Input: part model. Units: mm. Frame: model coordinates. Face numbers are marked on the shaded views. A direction names the side the tool comes from. Coordinates: 2 decimals unless noted, no trailing zeros. Write each loop counter-clockwise with the first axis right and the second up, starting at its lowest first coordinate (ties: lowest second). Pieces come first, ordered by that corner, then holes. Notation, with made-up numbers: M 17.25,80.25 L 54.25,80.25 A18 cw 54.25,97.25 Z; hole C 36,63.25 d2. An arc over 180 degrees is marked long. Use one line per item in the form item = value.
from build123d import *

# Parameters (mm, degrees)
SKETCH5_R                = 20
BOSS_EXTRUDE2_DEPTH      = 15
SKETCH6_W                = 30
SKETCH6_H                = 90
BOSS_EXTRUDE3_DEPTH      = 15
CIRPATTERN1_COUNT        = 3
BOSS_EXTRUDE4_DEPTH      = 5
FILLET1_R                = 3
SKETCH8_R                = 1
CUT_EXTRUDE1_DEPTH       = 16
SKETCH9_R                = 10
CUT_EXTRUDE2_DEPTH       = 10
CIRPATTERN4_COUNT        = 3
FILLET1_OF_CIRPATTERN4_R = 3
CIRPATTERN6_COUNT        = 3
CUT_EXTRUDE4_REACH       = 22
SKETCH11_R               = 2.875
SKETCH13_W               = 18
SKETCH13_H               = 18
CUT_EXTRUDE5_DEPTH       = 5
FILLET2_R                = 5
SKETCH14_R               = 5
CUT_EXTRUDE6_DEPTH       = 5


with BuildPart() as part:
    # Sketch5 → Boss-Extrude2 (new body)
    with BuildSketch(Plane(origin=(0, 0, 0), x_dir=(1, 0, 0), z_dir=(0, 1, 0))):
        Circle(SKETCH5_R)
    extrude(amount=BOSS_EXTRUDE2_DEPTH)

    # Sketch6 → Boss-Extrude3 (add)
    with BuildSketch(Plane(origin=(0, 0, 0), x_dir=(1, 0, 0), z_dir=(0, 1, 0))):
        with Locations((0, 45)):
            Rectangle(SKETCH6_W, SKETCH6_H)
    boss_extrude3 = extrude(amount=BOSS_EXTRUDE3_DEPTH)

    # CirPattern1: Boss-Extrude3 ×3 about axis
    cirpattern1_axis = Axis((0, 0, 0), (0, 1, 0))
    for i in range(1, CIRPATTERN1_COUNT):
        add(boss_extrude3.rotate(cirpattern1_axis, i * 360 / CIRPATTERN1_COUNT))

    # Sketch7 → Boss-Extrude4 (add)
    with BuildSketch(Plane(origin=(0, 15, 0), x_dir=(1, 0, 0), z_dir=(0, 1, 0))):
        Polygon((-13, 80), (13, 80), (13, 70.8), (5.25, 70.8), (5.25, 74.8), (-5.25, 74.8), (-5.25, 70.8), (-13, 70.8), align=None)
    boss_extrude4 = extrude(amount=BOSS_EXTRUDE4_DEPTH)

    # Fillet1
    fillet1_edges = [part.edges().sort_by_distance(p)[0] for p in [
        (-13, 17.5, -80),
        (-13, 17.5, -70.8),
        (13, 17.5, -70.8),
        (13, 17.5, -80),
    ]]
    fillet(fillet1_edges, radius=FILLET1_R)

    # Sketch8 → Cut-Extrude1 (cut, through all)
    with BuildSketch(Plane(origin=(0, 15, 0), x_dir=(1, 0, 0), z_dir=(0, 1, 0))):
        with Locations((0, 71.8)):
            Circle(SKETCH8_R)
    cut_extrude1 = extrude(amount=-CUT_EXTRUDE1_DEPTH, mode=Mode.SUBTRACT)

    # Sketch9 → Cut-Extrude2 (cut)
    with BuildSketch(Plane.XZ):
        with Locations((0, -71.8)):
            Circle(SKETCH9_R)
    cut_extrude2 = extrude(amount=-CUT_EXTRUDE2_DEPTH, mode=Mode.SUBTRACT)

    # CirPattern4: Boss-Extrude4 ×3 about axis
    cirpattern4_axis = Axis((0, 0, 0), (0, 1, 0))
    for i in range(1, CIRPATTERN4_COUNT):
        add(boss_extrude4.rotate(cirpattern4_axis, i * 360 / CIRPATTERN4_COUNT))

    # Fillet1 of CirPattern4
    fillet1_of_cirpattern4_edges = [part.edges().sort_by_distance(p)[0] for p in [
        (-62.782032303, 17.5, 51.258330249),
        (-54.814598588, 17.5, 46.658330249),
        (-67.814598588, 17.5, 24.141669751),
        (-75.782032303, 17.5, 28.741669751),
        (75.782032303, 17.5, 28.741669751),
        (67.814598588, 17.5, 24.141669751),
        (54.814598588, 17.5, 46.658330249),
        (62.782032303, 17.5, 51.258330249),
    ]]
    fillet(fillet1_of_cirpattern4_edges, radius=FILLET1_OF_CIRPATTERN4_R)

    # CirPattern6: Cut-Extrude1, Cut-Extrude2 ×3 about axis
    cirpattern6_axis = Axis((0, 0, 0), (0, 1, 0))
    for i in range(1, CIRPATTERN6_COUNT):
        add(cut_extrude1.rotate(cirpattern6_axis, i * 360 / CIRPATTERN6_COUNT), mode=Mode.SUBTRACT)
        add(cut_extrude2.rotate(cirpattern6_axis, i * 360 / CIRPATTERN6_COUNT), mode=Mode.SUBTRACT)

    # Sketch11 → Cut-Extrude4 (cut, up to next)
    with BuildSketch(Plane(origin=(0, 0, 0), x_dir=(1, 0, 0), z_dir=(0, 1, 0)), mode=Mode.PRIVATE) as cut_extrude4_sk1:
        Circle(SKETCH11_R)
    cut_extrude4_tool1 = extrude(cut_extrude4_sk1.sketch, amount=CUT_EXTRUDE4_REACH, mode=Mode.PRIVATE) & part.part
    add(cut_extrude4_tool1.solids().sort_by_distance((0, 0, 0))[0], mode=Mode.SUBTRACT)

    # Sketch13 → Cut-Extrude5 (cut)
    with BuildSketch(Plane.XZ):
        Rectangle(SKETCH13_W, SKETCH13_H)
    extrude(amount=-CUT_EXTRUDE5_DEPTH, mode=Mode.SUBTRACT)

    # Fillet2
    fillet2_edges = [part.edges().sort_by_distance(p)[0] for p in [
        (9, 2.5, 9),
        (9, 2.5, -9),
        (-9, 2.5, -9),
        (-9, 2.5, 9),
    ]]
    fillet(fillet2_edges, radius=FILLET2_R)

    # Sketch14 → Cut-Extrude6 (cut)
    with BuildSketch(Plane(origin=(0, 15, 0), x_dir=(1, 0, 0), z_dir=(0, 1, 0))):
        Circle(SKETCH14_R)
    extrude(amount=-CUT_EXTRUDE6_DEPTH, mode=Mode.SUBTRACT)


solid = part.part
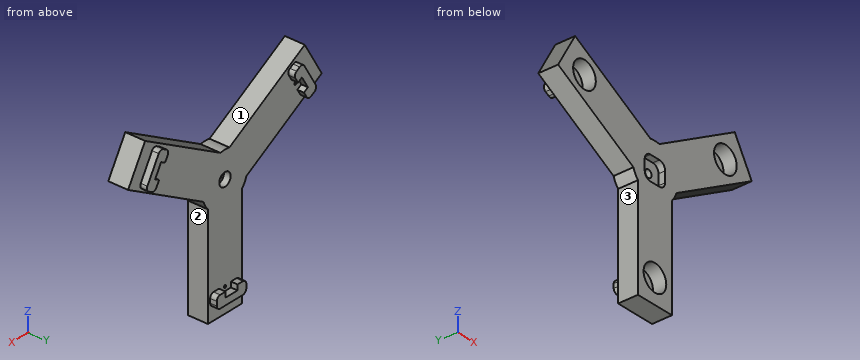
(1) Line query: probe 1 along Z at (x, y) = (0, 6) (3 decimals); probe 2 along Z at (x, y) = (0, 13.1); probe 3 along Y at (x, z) = (37, 37). Output: solid intervals per line, ascending.
Computed:
probe_1 = -90 to -81.8, -61.8 to -2.875, 2.875 to 20
probe_2 = -90 to -72.8, -70.8 to -5, 5 to 20
probe_3 = 0 to 15
(2) Section query D-D on x = 26. Return the cut outline in (y, z), plus the area to 3 significant figures.
Computed:
outline = M 0,-2.31 L 15,-2.31 L 15,32.33 L 0,32.33 Z
area = 520 mm^2
(3) Section query A-A on z = 0. Return the cut outline in (x, y) (3 decimals), plus the area to 3 significant figures.
Computed:
outline = M -30,0 L -9,0 L -9,5 L -2.875,5 L -2.875,10 L -5,10 L -5,15 L -30,15 Z; M 2.875,5 L 9,5 L 9,0 L 30,0 L 30,15 L 5,15 L 5,10 L 2.875,10 Z
area = 731 mm^2
(4) First-contact query: pin 1 Ø12 at (x, z) = (-37, 15.5) entering from +Y; pin 2 Ø1 at (y, z) = (11, 10.5) entering from -X; pin 3 Ø3 at (x, z) = (-62.18, 35.9) entering from -Y; pin 4 Ø1.8 at (x, z) = (62.18, 35.9) entering from +Y. Flat tips, straight axial feed; report the tip coordinate or a pass-through.
Computed:
pin_1 = 15
pin_2 = -49.05
pin_3 = 10
pin_4 = through
(5) Section query C-C on z = 22. Return the cut outline in (x, y), plus the area to 3 significant figures.
Computed:
outline = M -68.11,0 L -8.11,0 L -8.11,15 L -68.11,15 Z; M 8.11,0 L 68.11,0 L 68.11,15 L 8.11,15 Z
area = 1,800 mm^2
(6) Set-up query: the marked faces 1, 2 and 3. Return all of +Z, -Z, +X, -X, +Y, -Y with unobstructed straight access to the full face (end or side cutting, diameter ignored); none if empty.
Computed:
face_1 = +Z, +Y, -Y
face_2 = -Z, +X, +Y, -Y
face_3 = -Z, -X, +Y, -Y
(7) Section query B-B on y = 7.75. Return the cut outline in (x, z) (3 decimals).
Computed:
outline = M -85.442,32.01 L -18.956,-6.376 A20 ccw -15,-13.229 L -15,-90 L 15,-90 L 15,-13.229 A20 ccw 18.956,-6.376 L 85.442,32.01 L 70.442,57.99 L 3.956,19.605 A20 ccw -3.956,19.605 L -70.442,57.99 Z; hole C -62.181,35.9 d20; hole C 0,-71.8 d20; hole C 0,0 d5.75; hole C 62.181,35.9 d20
